For this review, take the finished solid that the model builds, in its own axes (mm). A direction names the side the tool comes from. Round coordinates to 2 decimals unless told otherwise and drop trailing zeros. Order: outer loops, then holes, each group sorted by start corner. A loop starts at its lowest first (then second) coordinate and runs counter-clockwise, first axis right, second up. Notation, with made-up numbers: (-22.75, 34.25) -> (1.25, 34.25) arc R24 cw to (1.25, 54.25) -> close; hole circle Ø7 at (-1, 27). An arc over 180 degrees is marked (long way). Answer in a Markdown table with one row per item.
```python
from build123d import *

# Parameters (mm, degrees)
SKETCH1_W           = 26
SKETCH1_H           = 12
BOSS_EXTRUDE1_DEPTH = 8
CUT_EXTRUDE1_DEPTH  = 28.856776554
SKETCH3_W           = 8.5
SKETCH3_H           = 10
CUT_EXTRUDE2_DEPTH  = 17.401219467
SKETCH4_R           = 1.5
CUT_EXTRUDE3_DEPTH  = 21.155644371
FILLET1_R           = 2
SKETCH5_R           = 1.5
CUT_EXTRUDE4_DEPTH  = 19.248287591


with BuildPart() as part:
    # Sketch1 → Boss-Extrude1 (new body)
    with BuildSketch(Plane.XY):
        Rectangle(SKETCH1_W, SKETCH1_H)
    extrude(amount=BOSS_EXTRUDE1_DEPTH)

    # Sketch2 → Cut-Extrude1 (cut, through all)
    with BuildSketch(Plane(origin=(13, 0, 0), x_dir=(0, 0, -1), z_dir=(1, 0, 0))):
        with BuildLine():
            Line((-8, 2), (-8, 7))
            Line((-8, 7), (0, 7))
            Line((0, 7), (0, 2))
            ThreePointArc((0, 2), (-4, 6), (-8, 2))
        make_face()
    extrude(amount=-CUT_EXTRUDE1_DEPTH, mode=Mode.SUBTRACT)

    # Sketch3 → Cut-Extrude2 (cut, through all)
    with BuildSketch(Plane.XY.offset(8)):
        with Locations((8.75, 1)):
            Rectangle(SKETCH3_W, SKETCH3_H)
        with Locations((-8.75, 1)):
            Rectangle(SKETCH3_W, SKETCH3_H)
    extrude(amount=-CUT_EXTRUDE2_DEPTH, mode=Mode.SUBTRACT)

    # Sketch4 → Cut-Extrude3 (cut, through all)
    with BuildSketch(Plane(origin=(4.5, 0, 0), x_dir=(0, 0, -1), z_dir=(1, 0, 0))):
        with Locations(Location((-4, 2, 0), (0, 0, 90))):
            Circle(SKETCH4_R)
    extrude(amount=-CUT_EXTRUDE3_DEPTH, mode=Mode.SUBTRACT)

    # Fillet1
    fillet1_edges = [part.edges().sort_by_distance(p)[0] for p in [
        (13, -5, 8),
        (13, -5, 0),
        (-13, -5, 8),
        (-13, -5, 0),
    ]]
    fillet(fillet1_edges, radius=FILLET1_R)

    # Sketch5 → Cut-Extrude4 (cut, through all)
    with BuildSketch(Plane(origin=(0, -4, 0), x_dir=(1, 0, 0), z_dir=(0, 1, 0))):
        with Locations(Location((-10, -4, 0), (0, 0, 180))):
            Circle(SKETCH5_R)
        with Locations(Location((10, -4, 0), (0, 0, 180))):
            Circle(SKETCH5_R)
    extrude(amount=-CUT_EXTRUDE4_DEPTH, mode=Mode.SUBTRACT)


solid = part.part
```
Q1. The part is to be moulded in two halves that separate along Z. For faces 4 (the face through (0, -3, 0)), 5 (the face through (0.06, 0.5, 4.07)), 6 (the face through (-8, -4, 4)), 7 (the face through (-8.5, -4.99, 4.07)), say which applies: +Z half, -Z half, draft (parallel to the pull), parting line (faces both ways), or undercut.
Answer key:
| item | result |
|---|---|
| face 4 | -Z half |
| face 5 | undercut |
| face 6 | draft |
| face 7 | undercut |
Q2. Take a section at D-D, the plane x = -5.5. Write out the cut boundary in (y, z), then the cut area to 3 significant figures.
Answer key:
| item | result |
|---|---|
| outline | (-6, 0) -> (-4, 0) -> (-4, 8) -> (-6, 8) -> close |
| area | 16.0 mm^2 |
Q3. Take a section at A-A, the plane x = 10. Write out the cut boundary in (y, z).
Answer key:
| item | result |
|---|---|
| outline | (-6, 0) -> (-4, 0) -> (-4, 2.5) -> (-6, 2.5) -> close; (-6, 5.5) -> (-4, 5.5) -> (-4, 8) -> (-6, 8) -> close |
Q4. Take a section at C-C, the plane z = 6.5. Write out the cut boundary in (x, y).
Answer key:
| item | result |
|---|---|
| outline | (-12.94, -6) -> (12.94, -6) -> (12.94, -4) -> (4.5, -4) -> (4.5, 5.12) -> (-4.5, 5.12) -> (-4.5, -4) -> (-12.94, -4) -> close |
Q5. Take a section at B-B, the plane y = 3. Write out the cut boundary in (x, z).
Answer key:
| item | result |
|---|---|
| outline | (-4.5, 0.13) -> (4.5, 0.13) -> (4.5, 2.88) -> (-4.5, 2.88) -> close; (-4.5, 5.12) -> (4.5, 5.12) -> (4.5, 7.87) -> (-4.5, 7.87) -> close |
Q6. Tool access review of faces 1 (the face through (-4.5, 0, 4)), 2 (the face through (8, -4, 4)), 3 (the face through (0, -6, 4)): name each direction out of +Z, -Z, +X, -X, +Y, -Y from which nothing blocks a thin tool from reaching the whole face with its end or side.
Answer key:
| item | result |
|---|---|
| face 1 | +Z, -Z, -X, +Y |
| face 2 | +Z, -Z, +X, +Y |
| face 3 | +Z, -Z, +X, -X, -Y |
Q7. To check wall thickness, follow probe 1 along Z at (x, y) = (-2, 2); probe 2 along X at (y, z) = (5, 3); probe 3 along Y at (x, z) = (11, 1). State the ranges of each line that lie inside material, in increasing order.
Answer key:
| item | result |
|---|---|
| probe 1 | z = 0 to 2.5, 5.5 to 8 |
| probe 2 | x = -4.5 to 4.5 |
| probe 3 | y = -6 to -4 |
Q8. Clearance check with flat-ended pins moving along their axes: pin 1 Ø4 at (y, z) = (0.5, 5.5) entering from -X; pin 2 Ø1 at (x, y) = (-2.5, 0) entering from -Z; pin 3 Ø4 at (x, y) = (-7.5, 2) entering from -Z. State where each tip first meets the part, or that it passes through.
Answer key:
| item | result |
|---|---|
| pin 1 | stops at x = -4.5 |
| pin 2 | stops at z = 0 |
| pin 3 | passes through |
